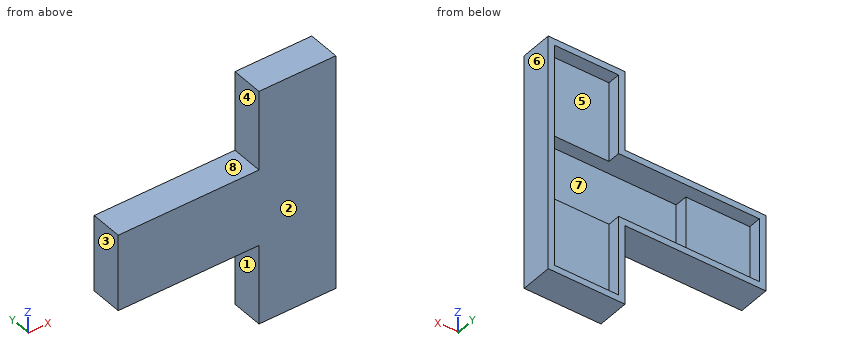
```python
from build123d import *

# Parameters (mm, degrees)
SKETCH_2_W           = 32
SKETCH_2_H           = 10
SKETCH_2_W_2         = 10
SKETCH_2_H_2         = 12.5
EXTRUDE_1_DEPTH      = 1
EXTRUDE_2_DEPTH      = 4
EXTRUDE_2_DEPTH_BACK = 1
SKETCH_4_W           = 10
SKETCH_4_H           = 10
SKETCH_4_H_2         = 12.5
EXTRUDE_3_DEPTH      = 2


with BuildPart() as part:
    # 草图2 → 凸台-拉伸1 (new body)
    with BuildSketch(Plane(origin=(0, 0, 0), x_dir=(1, 0, 0), z_dir=(0, 1, 0))):
        with Locations((-5, 0)):
            Rectangle(SKETCH_2_W, SKETCH_2_H)
        with Locations((6, 11.25)):
            Rectangle(SKETCH_2_W_2, SKETCH_2_H_2)
        with Locations((6, -11.25)):
            Rectangle(SKETCH_2_W_2, SKETCH_2_H_2)
    extrude(amount=EXTRUDE_1_DEPTH)

    # 草图3 → 凸台-拉伸2 (add, two sides)
    with BuildSketch(Plane(origin=(0, 1, 0), x_dir=(1, 0, 0), z_dir=(0, 1, 0))) as extrude_2_sk:
        Polygon((12, -18.5), (12, 18.5), (0, 18.5), (0, 6), (-22, 6), (-22, -6), (0, -6), (0, -18.5), align=None)
        Polygon((11, -17.5), (11, 17.5), (1, 17.5), (1, 5), (-21, 5), (-21, -5), (1, -5), (1, -17.5), align=None, mode=Mode.SUBTRACT)
    extrude(amount=EXTRUDE_2_DEPTH)
    extrude(extrude_2_sk.sketch, amount=-EXTRUDE_2_DEPTH_BACK)

    # 草图4 → 凸台-拉伸3 (add)
    with BuildSketch(Plane(origin=(0, 1, 0), x_dir=(1, 0, 0), z_dir=(0, 1, 0))):
        with Locations((-16, 0)):
            Rectangle(SKETCH_4_W, SKETCH_4_H)
        with Locations((6, 11.25)):
            Rectangle(SKETCH_4_W, SKETCH_4_H_2)
        with Locations((6, -11.25)):
            Rectangle(SKETCH_4_W, SKETCH_4_H_2)
    extrude(amount=EXTRUDE_3_DEPTH)


solid = part.part
```
CAD build for the part. Positions are in the model's coordinates, mm. Face numbers are marked on the shaded views. A direction names the side the tool comes from. Coordinates: 2 decimals unless noted, no trailing zeros. Write each loop counter-clockwise with the first axis right and the second up, starting at its lowest first coordinate (ties: lowest second). Pieces come first, ordered by that corner, then holes. Notation, with made-up numbers: (17.25, 23.25) -> (43.25, 23.25) arc R14 ccw to (43.25, 33.25) -> close; hole circle Ø2 at (88, 15.5). An arc over 180 degrees is marked (long way). Use CSV: the item, a comma, the result in double quotes. Start each with the question number.
Item 1: Two-plate mould, pull along X, no slides. Class the marked faces 6, 7 and 8: +X half, -X half, draft (parallel to the pull), parting line (faces both ways), or undercut.
Item 2: Band-saw the part on B-B, the plane z = 13. Write the cut outline in (x, y).
Item 3: Tool access for the marked faces 1, 2, 3, 4 and 5: list every direction of +Z, -Z, +X, -X, +Y, -Y with a clear straight run to the whole face (end or side of a thin tool).
Item 4: Band-saw the part on C-C, the plane x = -1. Write the cut outline in (y, z).
Item 5: Band-saw the part on D-D, the plane y = 4.2. Write the cut outline in (x, z), plus the area to 3 significant figures.
Item 6: Band-saw the part on A-A, the plane y = 1.6. Write the cut outline in (x, z).
Item 7: Drop flat-ended pins along their axis: P1, Ø1.5, axis at x = -6, y = 2, coming from the +Z side; P2, Ø3, axis at x = 7.5, z = 14, coming from the +Y side; P3, Ø6, axis at x = -9.5, z = -9.5, coming from the -Y side; P4, Ø1.2, axis at x = -10, y = 3.5, coming from the -Z side. Give the stop position or say it passes through.
Item 8: Wall check: probe 1 along Z at (x, y) = (-1.5, 1.9); probe 2 along X at (y, z) = (4.35, 14); probe 3 along X at (y, z) = (3.8, -3.5). Give the ranges that are in metal, low to high.
Response values:
1,face 6,"+X half"
1,face 7,"undercut"
1,face 8,"draft"
2,outline,"(0, 0) -> (12, 0) -> (12, 5) -> (11, 5) -> (11, 3) -> (1, 3) -> (1, 5) -> (0, 5) -> close"
3,face 1,"-Z, -X, +Y, -Y"
3,face 2,"+Z, -Z, +X, -X, -Y"
3,face 3,"+Z, -Z, -X, +Y, -Y"
3,face 4,"+Z, -X, +Y, -Y"
3,face 5,"+Y"
4,outline,"(0, -6) -> (5, -6) -> (5, -5) -> (1, -5) -> (1, 5) -> (5, 5) -> (5, 6) -> (0, 6) -> close"
5,outline,"(-22, -6) -> (0, -6) -> (0, -18.5) -> (12, -18.5) -> (12, 18.5) -> (0, 18.5) -> (0, 6) -> (-22, 6) -> close; hole (-21, -5) -> (1, -5) -> (1, -17.5) -> (11, -17.5) -> (11, 17.5) -> (1, 17.5) -> (1, 5) -> (-21, 5) -> close"
5,area,"138 mm2"
6,outline,"(-22, -6) -> (0, -6) -> (0, -18.5) -> (12, -18.5) -> (12, 18.5) -> (0, 18.5) -> (0, 6) -> (-22, 6) -> close; hole (-11, -5) -> (11, -5) -> (11, 5) -> (-11, 5) -> close"
7,P1,"stops at z = 6"
7,P2,"stops at y = 3"
7,P3,"passes through"
7,P4,"stops at z = -6"
8,probe 1,"z = -6 to -5, 5 to 6"
8,probe 2,"x = 0 to 1, 11 to 12"
8,probe 3,"x = -22 to -21, 11 to 12"
